Job drawing, mm, ordinate dimensions from the low corner. One solid piece. Coordinates: 2 decimals unless noted, no trailing zeros. Write each loop counter-clockwise with the first axis right and the second up, starting at its lowest first coordinate (ties: lowest second). Pieces come first, ordered by that corner, then holes. Notation, with made-up numbers: (-38, 81.25) - (0, 81.25) arc R8 ccw to (0, 96.25) - close; hole circle Ø10 at (61, 12). An arc over 180 degrees is marked (long way). Use one line per item in the form item = value. Start each with the question number.
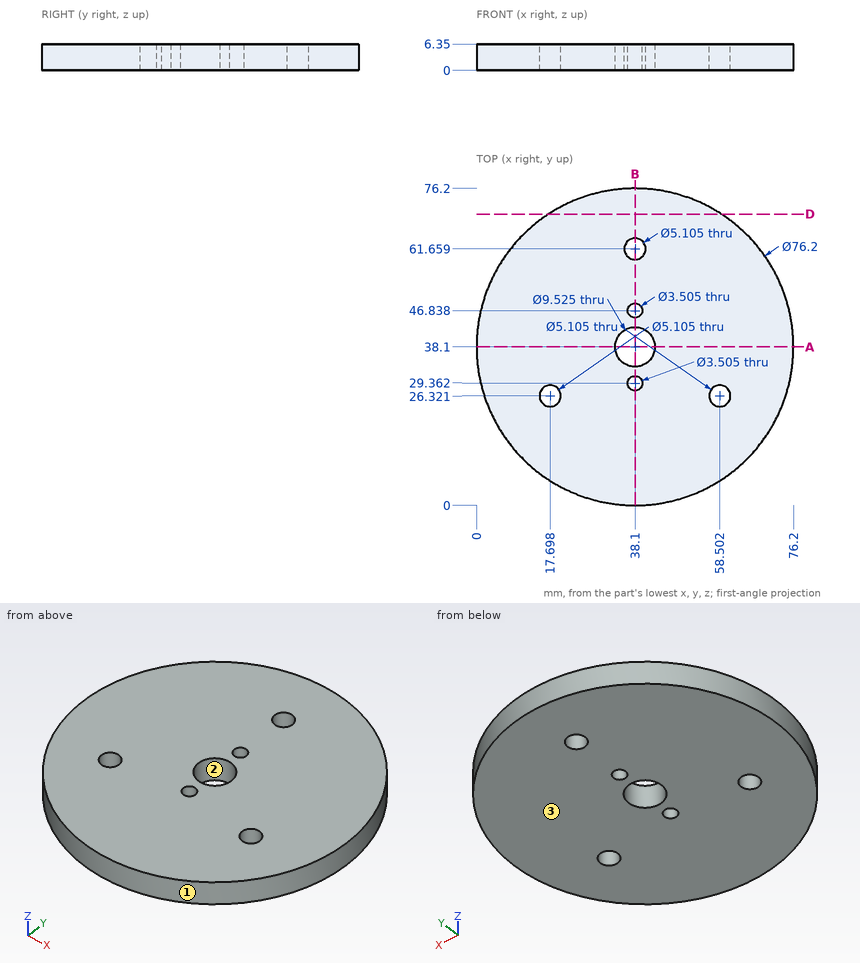
Q1. Drill centre lines: probe 1 along Y at (x, z) = (38.1, 4.75) (1 decimal); probe 2 along X at (y, z) = (24, 0.75) (1 decimal); probe 3 along Y at (x, z) = (59.5, 2.25). Where is each one in solid material? Low to high.
Q2. Slice it at D-D (y = 70). List the corners of the cut face in (x, z).
Q3. Slice it at B-B (x = 38.1). Count the separate pieces of the cut face and the enclosed holes in it.
Q4. Mould opens along Y. For the marked faces 1, 2 and 3 say: released by +Y, released by -Y, zero draft, split by the parting line, or undercut.
Q5. Slice it at A-A (y = 38.1). List the corners of the cut face in (x, z).
Q6. Pin check, flat tips, straight feed: P1, Ø2, axis at x = 38.1, y = 29.36, coming from the +Z side; P2, Ø1.5, axis at x = 55, z = 1, coming from the +Y side; P3, Ø1.5, axis at y = 54, z = 3, coming from the -X side; P4, Ø2, axis at y = 58.5, z = 4, coming from the +X side. Stop position of each tip, or through.
Solution:
q1.probe_1 = 0 to 27.6, 31.1 to 33.3, 42.9 to 45.1, 48.6 to 59.1, 64.2 to 76.2
q1.probe_2 = 2.7 to 16.6, 18.8 to 57.4, 59.6 to 73.5
q1.probe_3 = 6.58 to 23.97, 28.67 to 69.62
q2.outline = (17.27, 0) - (58.93, 0) - (58.93, 6.35) - (17.27, 6.35) - close
q3.separate_pieces = 5
q3.enclosed_holes = 0
q4.face_1 = split by the parting line
q4.face_2 = undercut
q4.face_3 = zero draft
q5.outline = (0, 0) - (33.34, 0) - (33.34, 6.35) - (0, 6.35) - close; (42.86, 0) - (76.2, 0) - (76.2, 6.35) - (42.86, 6.35) - close
q6.P1 = through
q6.P2 = 72.61
q6.P3 = 3.14
q6.P4 = 70.89
